For this review, take the finished solid that the model builds, in its own axes (mm). A direction names the side the tool comes from. Round coordinates to 2 decimals unless told otherwise and drop trailing zeros. Write each loop counter-clockwise with the first axis right and the second up, starting at its lowest first coordinate (ties: lowest second). Pieces come first, ordered by that corner, then holes. Notation, with made-up numbers: (18, 20.25) - (25, 20.25) arc R31 cw to (25, 51.25) - close; hole circle Ø1 at (-4.5, 68.5). An arc over 180 degrees is marked (long way). Answer in a Markdown table with one row per item. Add a question column.
from build123d import *

# Parameters (mm, degrees)
F0_W      = 30.48
F0_H      = 50.8
F2_DEPTH  = 7.62
F3_DEPTH  = 7.62
F4_DEPTH  = 5.461
F5_W      = 30.48
F5_H      = 7.62
F6_DEPTH  = 17.78
F8_DEPTH  = 7.62
F10_DEPTH = 7.62
F11_W     = 20.32
F11_H     = 3.81
F12_DEPTH = 6.35
F13_R     = 15.23999
F14_R     = 2.54


# Not quite as in the source:
# - a fillet or chamfer is up to 0.001 mm smaller than in the source, because OpenCascade refuses the exact size


with BuildPart() as f2:
    # F0 (on Front) → F2 (new body)
    with BuildSketch(Plane.XZ):
        Rectangle(F0_W, F0_H)
    extrude(amount=F2_DEPTH)

    # F1 (on face) → F3 (cut)
    with BuildSketch(Plane.XZ):
        with BuildLine():
            Line((4.7625, 0), (4.7625, 12.0856394065))
            ThreePointArc((4.7625, 12.0856394065), (0, 16.8481394065), (-4.7625, 12.0856394065))
            Line((-4.7625, 12.0856394065), (-4.7625, 0))
            ThreePointArc((-4.7625, 0), (-6.8685751798, -2.6488038051), (-7.62, -5.9483605935))
            ThreePointArc((-7.62, -5.9483605935), (0, -13.5683605935), (7.62, -5.9483605935))
            ThreePointArc((7.62, -5.9483605935), (6.8685751798, -2.6488038051), (4.7625, 0))
        make_face()
    extrude(amount=F3_DEPTH, mode=Mode.SUBTRACT)

    # F1 (on face) → F4 (cut)
    with BuildSketch(Plane.XZ):
        with BuildLine():
            Line((4.7625, 0), (4.7625, 12.0856394065))
            ThreePointArc((4.7625, 12.0856394065), (0, 16.8481394065), (-4.7625, 12.0856394065))
            Line((-4.7625, 12.0856394065), (-4.7625, 0))
            ThreePointArc((-4.7625, 0), (-6.8685751798, -2.6488038051), (-7.62, -5.9483605935))
            ThreePointArc((-7.62, -5.9483605935), (0, -13.5683605935), (7.62, -5.9483605935))
            ThreePointArc((7.62, -5.9483605935), (6.8685751798, -2.6488038051), (4.7625, 0))
        make_face()
        with BuildLine():
            ThreePointArc((-4.7625, 12.0856394065), (0, 16.8481394065), (4.7625, 12.0856394065))
            Line((4.7625, 12.0856394065), (4.7625, 0))
            ThreePointArc((4.7625, 0), (6.8685751798, -2.6488038051), (7.62, -5.9483605935))
            Line((7.62, -5.9483605935), (7.62, 12.0856394065))
            ThreePointArc((7.62, 12.0856394065), (0, 19.7056394065), (-7.62, 12.0856394065))
            Line((-7.62, 12.0856394065), (-7.62, -5.9483605935))
            ThreePointArc((-7.62, -5.9483605935), (-6.8685751798, -2.6488038051), (-4.7625, 0))
            Line((-4.7625, 0), (-4.7625, 12.0856394065))
        make_face()
    extrude(amount=F4_DEPTH, mode=Mode.SUBTRACT)

    # F5 (on face) → F6 (join)
    with BuildSketch(Plane(origin=(0, 0, 0), x_dir=(-1, 0, 0), z_dir=(0, 1, 0))):
        with Locations((0, -21.59)):
            Rectangle(F5_W, F5_H)
    extrude(amount=F6_DEPTH)

    # F7 (on face) → F8 (join)
    with BuildSketch(Plane.YZ.offset(15.24)):
        with BuildLine():
            ThreePointArc((11.0238203779, -17.78), (3.2923822905, -14.1798622678), (0, -6.3124392182))
            Line((0, -6.3124392182), (0, -17.78))
            Line((0, -17.78), (11.0238203779, -17.78))
        make_face()
    extrude(amount=-F8_DEPTH)

    # F9 (on face) → F10 (join)
    with BuildSketch(Plane(origin=(-15.24, 0, 0), x_dir=(0, -1, 0), z_dir=(-1, 0, 0))):
        with BuildLine():
            Line((-11.0238286, -17.78), (0, -17.78))
            Line((0, -17.78), (0, -5.9952606229))
            ThreePointArc((0, -5.9952606229), (-3.1855434206, -14.0637933146), (-11.0238286, -17.78))
        make_face()
    extrude(amount=-F10_DEPTH)

    # F11 (on face) → F12 (cut)
    with BuildSketch(Plane.XZ.offset(7.62)):
        with Locations((0, -21.59)):
            Rectangle(F11_W, F11_H)
    extrude(amount=-F12_DEPTH, mode=Mode.SUBTRACT)

    # F13 (radius 15.24 in the source; OpenCascade refuses exactly that, so slightly less here)
    f13_edges = [f2.edges().sort_by_distance(p)[0] for p in [
        (15.24, -3.81, 25.4),
        (-15.24, -3.81, 25.4),
    ]]
    fillet(f13_edges, radius=F13_R)

    # F14
    f14_edges = [f2.edges().sort_by_distance(p)[0] for p in [
        (4.7625, -6.5405, 0),
        (-4.7625, -6.5405, 0),
    ]]
    fillet(f14_edges, radius=F14_R)


solid = f2.part
Q1. To check wall thickness, follow probe 1 along X at (y, z) = (0.25, -10); probe 2 along Z at (x, y) = (5, -1.75) (3 decimals); probe 3 along Z at (x, y) = (-8, 14.75). State the ranges of each line that lie inside material, in increasing order.
Q2. Add section B-B on x = -7. State the section outline as (y, z) points (3 decimals).
Q3. Add section C-C on y = 1.5. State the section outline as (x, z) points, then the cut area to 3 significant figures.
Q4. Insertion check: pin 1 Ø1.9 at (x, z) = (4.5, -21) entering from -Y; pin 2 Ø17 at (x, z) = (-2, 12.5) entering from +Y; pin 3 Ø8 at (x, y) = (8, 14) entering from +Z. Each pin has a flat end and moves straight along its axis. Give the tip position at first contact, or say it passes through.
Q5. Draft analysis for pull direction X (two halves, no side actions). For faces 5 (the face through (0, 17.78, -22)), 6 (the face through (4.762, -7, 7)), state which applies: released by +X, released by -X, zero draft, split by the parting line, or undercut.
Q6. Add section A-A on z = 9. State the section outline as (x, y) points.
Q7. Add section D-D on z = -21.5. State the section outline as (x, y) points.
Q8. Tool access review of faces 1 (the face through (-4.953, -6.556, 0.15)), 2 (the face through (-7.62, 3, -15)), 3 (the face through (-7.62, -3, 3)), 4 (the face through (0, -4, -19.685)): name each direction out of +Z, -Z, +X, -X, +Y, -Y from which nothing blocks a thin tool from reaching the whole face with its end or side.
Answer sheet:
| question | item | result |
|---|---|---|
| 1 | probe 1 | x = -15.24 to -7.62, 7.62 to 15.24 |
| 1 | probe 2 | z = -25.4 to -23.495, -19.685 to -11.699, 17.836 to 24.556 |
| 1 | probe 3 | z = -25.4 to -17.78 |
| 2 | outline | (-7.62, -25.4) - (17.78, -25.4) - (17.78, -17.78) - (0, -17.78) - (0, -8.959) - (-7.62, -8.959) - (-7.62, -19.685) - (-1.27, -19.685) - (-1.27, -23.495) - (-7.62, -23.495) - close; (-7.62, -2.938) - (-5.461, -2.938) - (-5.461, 15.096) - (0, 15.096) - (0, 23.697) - (-7.62, 23.697) - close |
| 3 | outline | (-15.24, -25.4) - (15.24, -25.4) - (15.24, -11.76) - (7.62, -11.76) - (7.62, -17.78) - (-7.62, -17.78) - (-7.62, -11.76) - (-15.24, -11.76) - close |
| 3 | area | 324 mm² |
| 4 | pin 1 | stops at y = -1.27 |
| 4 | pin 2 | stops at y = 0 |
| 4 | pin 3 | stops at z = -17.67 |
| 5 | face 5 | zero draft |
| 5 | face 6 | undercut |
| 6 | outline | (-15.24, -7.62) - (-4.76, -7.62) - (-4.76, -5.46) - (-7.62, -5.46) - (-7.62, 0) - (-15.24, 0) - close; (4.76, -7.62) - (15.24, -7.62) - (15.24, 0) - (7.62, 0) - (7.62, -5.46) - (4.76, -5.46) - close |
| 7 | outline | (-15.24, -7.62) - (-10.16, -7.62) - (-10.16, -1.27) - (10.16, -1.27) - (10.16, -7.62) - (15.24, -7.62) - (15.24, 17.78) - (-15.24, 17.78) - close |
| 8 | face 1 | +Y, -Y |
| 8 | face 2 | +Z, +Y |
| 8 | face 3 | +Y |
| 8 | face 4 | -Y |
